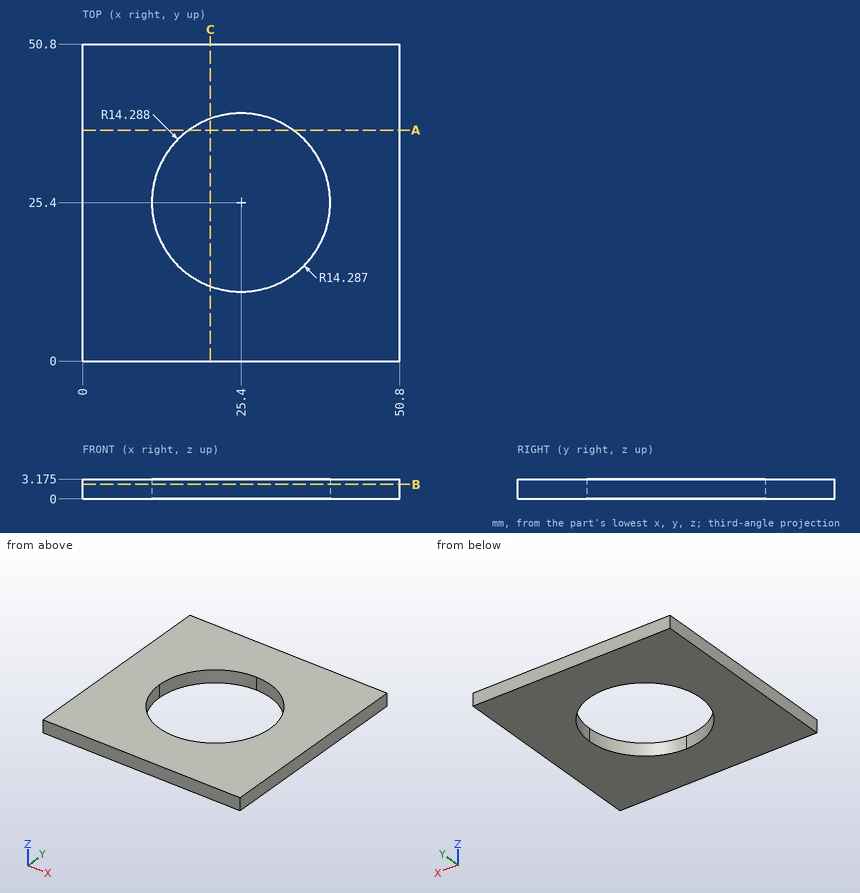
Print and shaded views of the part. All mm, measured from the part's lowest x, y and z. Coordinates: 2 decimals unless noted, no trailing zeros. Order: outer loops, then holes, each group sorted by start corner. A loop starts at its lowest first (then second) coordinate and runs counter-clockwise, first axis right, second up. Notation, with made-up numbers: M 68,18.5 L 80,18.5 A28 cw 80,45.5 Z; hole C 72.25,61.25 d2. An arc over 180 degrees is marked long. Write each question's results on one line, items separated by ' | '. Start each with the question number.
Q1. Cut at C-C (x = 20.5). List the corners of the cut face in (y, z) (1 decimal).
Q2. Cut at B-B (z = 2.3). List the corners of the cut face in (x, y) (1 decimal).
Q3. Cut at A-A (y = 37). List the corners of the cut face in (x, z) (1 decimal).
Q4. Drill centre lines: probe 1 along X at (y, z) = (18.5, 0.85); probe 2 along X at (y, z) = (27.5, 0.2); probe 3 along Y at (x, z) = (20.5, 2.9). Where is each one in solid material? Low to high. Write a range as from..to.
Found:
1) outline: M 0,0 L 12,0 L 12,3.2 L 0,3.2 Z; M 38.8,0 L 50.8,0 L 50.8,3.2 L 38.8,3.2 Z
2) outline: M 0,0 L 50.8,0 L 50.8,50.8 L 0,50.8 Z; hole C 25.4,25.4 d28.6
3) outline: M 0,0 L 17.1,0 L 17.1,3.2 L 0,3.2 Z; M 33.7,0 L 50.8,0 L 50.8,3.2 L 33.7,3.2 Z
4) probe 1: 0..12.89, 37.91..50.8 | probe 2: 0..11.27, 39.53..50.8 | probe 3: 0..11.98, 38.82..50.8
